```python
from build123d import *

# Parameters (mm, degrees)
EXTRUDE_1_DEPTH     = 8
CUT_EXTRUDE_1_REACH = 34.404
SKETCH_4_R          = 1.5
EXTRUDE_START       = 1
SKETCH_5_R          = 2
SKETCH_5_R_2        = 1.5
EXTRUDE_2_DEPTH     = 1
SKETCH_6_R          = 2
SKETCH_6_R_2        = 1.5
EXTRUDE_3_DEPTH     = 1
FILLET_1_R          = 1
FILLET_2_R          = 1
SKETCH_7_R          = 1.5
CUT_EXTRUDE_2_DEPTH = 5
CUT_EXTRUDE_3_DEPTH = 2


with BuildPart() as part:
    # Эскиз3 → Бобышка-Вытянуть1 (new body)
    with BuildSketch(Plane(origin=(0, 0, 0), x_dir=(0, 0, -1), z_dir=(1, 0, 0))):
        Polygon((0, 0), (25, 0), (25, 4), (5, 4), (5, 15), (25, 15), (25, 19), (0, 19), align=None)
    extrude(amount=EXTRUDE_1_DEPTH)

    # Вырез-Вытянуть1: up to this face of the body (flat: up to its plane)
    cut_extrude_1_end = Plane(part.part.faces().sort_by_distance((4, 0, -12.5))[0])
    # Эскиз4 → Вырез-Вытянуть1 (cut, up to the picked face)
    with BuildSketch(Plane(origin=(0, 19, 0), x_dir=(1, 0, 0), z_dir=(0, 1, 0)), mode=Mode.PRIVATE) as cut_extrude_1_sk1:
        with Locations(Location((4, 19, 0), (0, 0, 270))):
            Circle(SKETCH_4_R)
    cut_extrude_1_tool1 = split(extrude(cut_extrude_1_sk1.sketch, amount=-CUT_EXTRUDE_1_REACH, mode=Mode.PRIVATE), bisect_by=cut_extrude_1_end, keep=Keep.BOTH, mode=Mode.PRIVATE)
    add(cut_extrude_1_tool1.solids().sort_by(Axis((4, 19, -19), (0, -1, 0)))[0], mode=Mode.SUBTRACT)

    # Эскиз5 → Бобышка-Вытянуть2 (add)
    with BuildSketch(Plane(origin=(0, 4, 0), x_dir=(1, 0, 0), z_dir=(0, 1, 0)).offset(EXTRUDE_START)):
        with Locations(Location((4, 19, 0), (0, 0, 90))):
            Circle(SKETCH_5_R)
        with Locations(Location((4, 19, 0), (0, 0, 270))):
            Circle(SKETCH_5_R_2, mode=Mode.SUBTRACT)
    extrude(amount=-EXTRUDE_2_DEPTH)

    # Эскиз6 → Бобышка-Вытянуть3 (add)
    with BuildSketch(Plane(origin=(0, 15, 0), x_dir=(-1, 0, 0), z_dir=(0, -1, 0))):
        with Locations(Location((-4, 19, 0), (0, 0, 90))):
            Circle(SKETCH_6_R)
        with Locations(Location((-4, 19, 0), (0, 0, 270))):
            Circle(SKETCH_6_R_2, mode=Mode.SUBTRACT)
    extrude(amount=EXTRUDE_3_DEPTH)

    # Скругление1
    fillet_1_edges = [part.edges().sort_by_distance(p)[0] for p in [
        (4, 4, -17),
    ]]
    fillet(fillet_1_edges, radius=FILLET_1_R - 0.0001)  # a hair under: the kernel refuses the full size

    # Скругление2
    fillet_2_edges = [part.edges().sort_by_distance(p)[0] for p in [
        (4, 15, -17),
    ]]
    fillet(fillet_2_edges, radius=FILLET_2_R - 0.0001)  # a hair under: the kernel refuses the full size

    # Эскиз7 → Вырез-Вытянуть2 (cut)
    with BuildSketch(Plane(origin=(0, 0, -5), x_dir=(-1, 0, 0), z_dir=(0, 0, -1))):
        with Locations((-4, 9.5)):
            Circle(SKETCH_7_R)
    extrude(amount=-CUT_EXTRUDE_2_DEPTH, mode=Mode.SUBTRACT)

    # Эскиз9 → Вырез-Вытянуть3 (cut)
    with BuildSketch(Plane(origin=(0, 0, -5), x_dir=(-1, 0, 0), z_dir=(0, 0, -1))):
        Polygon((-1.264118223, 11.111919426), (-4.028022284, 12.675302834), (-6.763904061, 11.063383407), (-6.735881777, 7.888080574), (-3.971977716, 6.324697166), (-1.236095939, 7.936616593), align=None)
    extrude(amount=-CUT_EXTRUDE_3_DEPTH, mode=Mode.SUBTRACT)


solid = part.part
```
The listing builds one solid part. Answer for the finished solid, in the listing's coordinates (mm). A direction names the side the tool comes from. Coordinates: 2 decimals unless noted, no trailing zeros. Write each loop counter-clockwise with the first axis right and the second up, starting at its lowest first coordinate (ties: lowest second). Pieces come first, ordered by that corner, then holes. Notation, with made-up numbers: M -21,-17.5 L -11,-17.5 A27 cw -11,12.5 Z; hole C 41.25,8.25 d1. An arc over 180 degrees is marked long. Use a Markdown table: item, result. Add a question column.
1. Section B-B (z = -7) is taken. Give the vertices of the cut face in (x, y), plus the area to 3 significant figures.
2. Which of the six approach directions +Z, -Z, +X, -X, +Y, -Y give full straight-line access (tool end or side, diameter ignored) to faces 5 (the flat face through (2.627, 11.883, -4.014)), 6 (the flat face through (4, 0, -12)), 7 (the flat face through (6, 12, -5))?
3. For a pull along X with two mould halves and no side action, classify faces 1 (the flat face through (2.62, 7.12, -4.01)), 2 (the flat face through (4, 4, -15)), 3 (the flat face through (8, 10, -4)), 4 (the flat face through (5.373, 7.117, -4.014)) as +X half, -X half, draft (parallel to the pull), parting line (faces both ways), or undercut.
4. Straight lines are drawn through the part: line 1 along Z through (x, y) = (4, 16.9); line 2 along Y through (x, z) = (5, -9.75); line 3 along X through (y, z) = (3.2, -19). For each, find the intervals that lie inside material, in ascending order. Write a range as [from, to].
5. Given P1, Ø4, axis at x = 4, y = 11.5, coming from the -Z side, flat-ended and moving along its own axis, determine where the tip first touches the part or whether it passes through.
6. Section D-D (y = 8.5) is taken. Give the vertices of the cut face in (x, z), plus the area to 3 significant figures.
7. Section C-C (y = 2.25) is taken. Give the vertices of the cut face in (x, z), plus the area to 3 significant figures.
8. Section A-A (z = -19) is taken. Count the separate pieces of the cut face and the enclosed holes in it, plus the area to 3 significant figures.
Data:
| question | item | result |
|---|---|---|
| 1 | outline | M 0,0 L 8,0 L 8,4 L 0,4 Z; M 0,15 L 8,15 L 8,19 L 0,19 Z |
| 1 | area | 64.0 mm2 |
| 2 | face 5 | -Z |
| 2 | face 6 | +Z, -Z, +X, -X, -Y |
| 2 | face 7 | +X, -X |
| 3 | face 1 | undercut |
| 3 | face 2 | draft |
| 3 | face 3 | +X half |
| 3 | face 4 | undercut |
| 4 | line 1 | z = [-25, -20.5], [-17.5, 0] |
| 4 | line 2 | y = [0, 4], [15, 19] |
| 4 | line 3 | x = [0, 2.5], [5.5, 8] |
| 5 | P1 | stops at z = -5 |
| 6 | outline | M 0,-5 L 1.24,-5 L 1.24,-3 L 2.88,-3 L 2.88,0 L 0,0 Z; M 5.12,-3 L 6.74,-3 L 6.74,-5 L 8,-5 L 8,0 L 5.12,0 Z |
| 6 | area | 22.3 mm2 |
| 7 | outline | M 0,-25 L 8,-25 L 8,0 L 0,0 Z; hole C 4,-19 d3 |
| 7 | area | 193 mm2 |
| 8 | separate pieces | 4 |
| 8 | enclosed holes | 0 |
| 8 | area | 42.9 mm2 |
